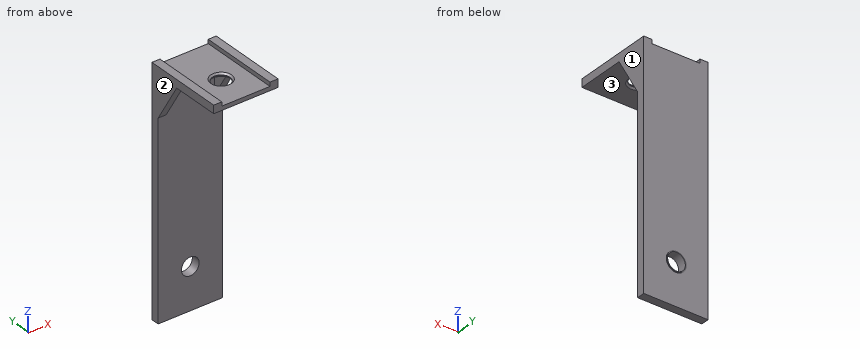
```python
from build123d import *

# Parameters (mm, degrees)
DODANIE_WYCI_GNI_CIE1_DEPTH = 40
SZKIC2_W                    = 30
SZKIC2_H                    = 2.5
WYTNIJ_WYCI_GNI_CIE1_DEPTH  = 164.095064303
EBRO3_START                 = -5
EBRO3_DEPTH                 = 5
SZKIC4_R                    = 5.5
WYTNIJ_WYCI_GNI_CIE2_DEPTH  = 10
SFAZOWANIE1_SIZE            = 1
WYTNIJ_WYCI_GNI_CIE3_DEPTH  = 10
DODANIE_WYCI_GNI_CIE2_START = 0.5
SZKIC6_R                    = 6
SZKIC6_R_2                  = 5.5
DODANIE_WYCI_GNI_CIE2_DEPTH = 0.5


# Read off the part's stored shape, not the designer's step: Żebro3
with BuildPart() as part:
    # Szkic1 → Dodanie-wyciągnięcie1 (new body)
    with BuildSketch(Plane(origin=(0, 0, 0), x_dir=(0, 0, -1), z_dir=(1, 0, 0))):
        Polygon((0, 0), (0, 50), (150, 50), (150, 45), (5, 45), (5, 0), align=None)
    extrude(amount=DODANIE_WYCI_GNI_CIE1_DEPTH)

    # Szkic2 → Wytnij-wyciągnięcie1 (cut, through all)
    with BuildSketch(Plane(origin=(0, 50, 0), x_dir=(1, 0, 0), z_dir=(0, 1, 0))):
        with Locations((20, 1.25)):
            Rectangle(SZKIC2_W, SZKIC2_H)
    extrude(amount=-WYTNIJ_WYCI_GNI_CIE1_DEPTH, mode=Mode.SUBTRACT)

    # Żebro3 outline → Żebro3 (add)
    with BuildSketch(Plane(origin=(40, 0, 0), x_dir=(0, 0, -1), z_dir=(1, 0, 0)).offset(EBRO3_START)):
        Polygon((5, 30), (30, 45), (5, 45), align=None)
    ebro3 = extrude(amount=EBRO3_DEPTH)

    # Lustro1: Żebro3 across plane
    add(ebro3.mirror(Plane(origin=(20, 0, 0), x_dir=(0, 0, 1), z_dir=(1, 0, 0))))

    # Szkic4 → Wytnij-wyciągnięcie2 (cut)
    with BuildSketch(Plane(origin=(0, 0, -5), x_dir=(-1, 0, 0), z_dir=(0, 0, -1))):
        with Locations((-20, 20)):
            Circle(SZKIC4_R)
    extrude(amount=-WYTNIJ_WYCI_GNI_CIE2_DEPTH, mode=Mode.SUBTRACT)

    # Sfazowanie1
    sfazowanie1_edges = [part.edges().sort_by_distance(p)[0] for p in [
        (25.5, 20, -2.5),
        (25.5, 20, -5),
    ]]
    chamfer(sfazowanie1_edges, length=SFAZOWANIE1_SIZE)

    # Szkic5 → Wytnij-wyciągnięcie3 (cut)
    with BuildSketch(Plane(origin=(0, 50, 0), x_dir=(1, 0, 0), z_dir=(0, 1, 0))):
        with BuildLine():
            ThreePointArc((20, 129.597336258), (14.5, 124.097336258), (20, 118.597336258))
            Line((20, 118.597336258), (20, 129.597336258))
        make_face()
        with BuildLine():
            Line((20, 129.597336258), (20, 118.597336258))
            ThreePointArc((20, 118.597336258), (23.889087297, 120.208248962), (25.5, 124.097336258))
            ThreePointArc((25.5, 124.097336258), (23.889087297, 127.986423555), (20, 129.597336258))
        make_face()
    extrude(amount=-WYTNIJ_WYCI_GNI_CIE3_DEPTH, mode=Mode.SUBTRACT)

    # Szkic6 → Dodanie-wyciągnięcie2 (add)
    with BuildSketch(Plane(origin=(0, 50, 0), x_dir=(1, 0, 0), z_dir=(0, 1, 0)).offset(DODANIE_WYCI_GNI_CIE2_START)):
        with Locations(Location((20, 124.097336258, 0), (0, 0, 270))):
            Circle(SZKIC6_R)
        with Locations(Location((20, 124.097336258, 0), (0, 0, 270))):
            Circle(SZKIC6_R_2, mode=Mode.SUBTRACT)
    extrude(amount=-DODANIE_WYCI_GNI_CIE2_DEPTH)


solid = part.part
```
CAD build for the part. Positions are in the model's coordinates, mm. Face numbers are marked on the shaded views. Round coordinates to 2 decimals unless told otherwise and drop trailing zeros. Order: outer loops, then holes, each group sorted by start corner. A loop starts at its lowest first (then second) coordinate and runs counter-clockwise, first axis right, second up.
Item 1: Saw through at A-A on y = 20. Write the cut outline in (x, z), then the cut area to 3 significant figures.
Item 2: Probe line 1 along Y through (x, z) = (20, -3.55); line 2 along Z through (x, y) = (20, 48.25); line 3 along Z through (x, y) = (26, 30.5). List the from-to ranges inside material, lowest first.
Item 3: Saw through at B-B on x = 32.5. Write the cut outline in (y, z).
Item 4: Mould opens along X. For the marked faces 1, 2 and 3 say: pulls with the +X half, pulls with the -X half, needs draft (parallel to the pull), parting line crosses it, or undercut.
Item 5: Saw through at C-C on z = -83.5. Write the cut outline in (x, y), then the cut area to 3 significant figures.
Item 6: Pin check, flat tips, straight feed: pin 1 (0.8 mm diameter, centred on y = 27, z = -1, fed in from -X); pin 2 (6 mm diameter, centred on x = 29, y = 26, fed in from +Z); pin 3 (4 mm diameter, centred on x = 32.5, y = 19.5, fed in from -Z). Stop position of each tip, or through.
Reported:
1. outline: (0, -5) - (13.5, -5) - (14.5, -4) - (14.5, -3.5) - (13.5, -2.5) - (5, -2.5) - (5, 0) - (0, 0) - close; (25.5, -4) - (26.5, -5) - (40, -5) - (40, 0) - (35, 0) - (35, -2.5) - (26.5, -2.5) - (25.5, -3.5) - close
1. area: 95.5 mm2
2. line 1: y = 0 to 14.5, 25.5 to 50
2. line 2: z = -150 to -129.6, -118.6 to -2.5
2. line 3: z = -5 to -2.5
3. outline: (0, -5) - (45, -5) - (45, -150) - (50, -150) - (50, -2.5) - (0, -2.5) - close
4. face 1: pulls with the +X half
4. face 2: pulls with the -X half
4. face 3: undercut
5. outline: (0, 45) - (40, 45) - (40, 50) - (0, 50) - close
5. area: 200 mm2
6. pin 1: stops at x = 0
6. pin 2: stops at z = -2.5
6. pin 3: stops at z = -5
